from build123d import *

# Parameters (mm, degrees)
F0_R     = 16.2722693288
F0_R_2   = 9.1584338909
F1_DEPTH = 25


# Not quite as in the source:
# - the program builds the solid bodies; features that only make, move or delete a surface that nothing else refers to are left out


with BuildPart() as f1:
    # F0 (on Front) → F1 (new body)
    with BuildSketch(Plane.XZ):
        with BuildLine():
            Line((-40.7540334754, 34.5627303773), (-50.2872206271, 35.8533678809))
            ThreePointArc((-50.2872206271, 35.8533678809), (-86.140588508, 0), (-50.2872206271, -35.8533678809))
            Line((-50.2872206271, -35.8533678809), (-40.7540334754, -34.5627303773))
            ThreePointArc((-40.7540334754, -34.5627303773), (-21.7630128867, -21.721730161), (-14.4338527462, 0))
            ThreePointArc((-14.4338527462, 0), (-21.7630128867, 21.721730161), (-40.7540334754, 34.5627303773))
        make_face()
        with Locations((-50.2872206271, 0)):
            Circle(F0_R, mode=Mode.SUBTRACT)
        with BuildLine():
            Line((58.6960054934, 21.0988228735), (-40.7540334754, 34.5627303773))
            ThreePointArc((-40.7540334754, 34.5627303773), (-21.7630128867, 21.721730161), (-14.4338527462, 0))
            ThreePointArc((-14.4338527462, 0), (-21.7630128867, -21.721730161), (-40.7540334754, -34.5627303773))
            Line((-40.7540334754, -34.5627303773), (58.6960054934, -21.0988228735))
            ThreePointArc((58.6960054934, -21.0988228735), (37.59718262, 0), (58.6960054934, 21.0988228735))
        make_face()
        with BuildLine():
            ThreePointArc((79.7948283669, 0), (73.6151262223, 14.9191207289), (58.6960054934, 21.0988228735))
            ThreePointArc((58.6960054934, 21.0988228735), (37.59718262, 0), (58.6960054934, -21.0988228735))
            ThreePointArc((58.6960054934, -21.0988228735), (73.6151262223, -14.9191207289), (79.7948283669, 0))
        make_face()
        with Locations((58.6960054934, 0)):
            Circle(F0_R_2, mode=Mode.SUBTRACT)
    extrude(amount=-F1_DEPTH)


solid = f1.part
Work out the finished part from the listing and answer in its coordinate system (mm). Coordinates: 2 decimals unless noted, no trailing zeros. Write each loop counter-clockwise with the first axis right and the second up, starting at its lowest first coordinate (ties: lowest second). Pieces come first, ordered by that corner, then holes. Notation, with made-up numbers: M 67,57.25 L 112,57.25 A20 ccw 112,68.25 Z; hole C 73,55.5 d2. An arc over 180 degrees is marked long. Answer as CSV lines item,"result". Start each with the question number.
Item 1: Section C-C on x = -47.5 is taken. Write down the section's boundary in (y, z).
Item 2: Section D-D on z = -27.5 is taken. Write down the section's boundary in (x, y), and give its area (3 significant figures).
Item 3: Consider L1, parallel to Z at x = 58.5, y = 7.25; L2, parallel to X at y = 7, z = -8; L3, parallel to X at y = 6.5, z = -3. Determine where each line is inside the solid, lowest interval first.
Item 4: Section B-B on x = 53 is taken. Write down the section's boundary in (y, z), and give its area (3 significant figures).
Item 5: Section A-A on y = 23 is taken. Write down the section's boundary in (x, z), and give its area (3 significant figures).
Item 6: Flat-ended cylindrical pins translate along their axes: P1, Ø5, axis at x = 59.5, z = 6, coming from the +Y side; P2, Ø12, axis at y = 3.5, z = -15.5, coming from the -X side; P3, Ø1, axis at x = -51.5, y = 3, coming from the +Z side; P4, Ø12, axis at x = -44.5, z = 10.5, coming from the +Y side. Find the tip coordinate at first contact, or state that the pin passes through.
Item 7: Determine the mould class of faces 1 (the face through (67.43, 12.32, 2.75)), 2 (the face through (-86.13, 12.32, 0.79)), 3 (the face through (-4, 25, 1)) for opening direction Z: released by +Z, released by -Z, zero draft, split by the parting line, or undercut.
Checks:
1,outline,"M 0,-35.48 L 25,-35.48 L 25,-16.03 L 0,-16.03 Z; M 0,16.03 L 25,16.03 L 25,35.48 L 0,35.48 Z"
2,outline,"M -73.29,0 L 11.41,0 L 11.41,25 L -73.29,25 Z"
2,area,"2,120 mm²"
3,L1,"z = -21.13 to -9.16, 9.16 to 21.13"
3,L2,"x = -85.24 to -64.46, -36.12 to 54.24, 63.15 to 78.22"
3,L3,"x = -86.01 to -66.28, -34.29 to 50.04, 67.35 to 79.58"
4,outline,"M 0,-21.87 L 25,-21.87 L 25,-7.17 L 0,-7.17 Z; M 0,7.17 L 25,7.17 L 25,21.87 L 0,21.87 Z"
4,area,"735 mm²"
5,outline,"M -50.29,-35.85 L 58.7,-21.1 A21.1 ccw 58.7,21.1 L -50.29,35.85 A35.85 ccw Z; hole C -50.29,0 d32.54; hole C 58.7,0 d18.32"
5,area,"7,830 mm²"
6,P1,"passes through"
6,P2,"stops at x = -84.86"
6,P3,"stops at z = 35.85"
6,P4,"stops at y = 25"
7,face 1,"undercut"
7,face 2,"split by the parting line"
7,face 3,"zero draft"
